```python
from build123d import *

# Parameters (mm, degrees)
SKETCH_1_R               = 150.987526818
SKETCH_1_R_2             = 138.21111966
EXTRUDE_1_DEPTH          = 15
FILLET_1_R               = 2
SKETCH_2_R               = 10
CUT_EXTRUDE_1_DEPTH      = 15
PATTERN_CIRCULAR_1_COUNT = 6


with BuildPart() as part:
    # Эскиз1 → Бобышка-Вытянуть1 (new body)
    with BuildSketch(Plane(origin=(0, 0, 0), x_dir=(1, 0, 0), z_dir=(0, 1, 0))):
        with Locations(Location((0, 0, 0), (0, 0, 270))):
            Circle(SKETCH_1_R)
        with Locations(Location((0, 0, 0), (0, 0, 270))):
            Circle(SKETCH_1_R_2, mode=Mode.SUBTRACT)
    extrude(amount=EXTRUDE_1_DEPTH)

    # Скругление1
    fillet_1_edges = [part.edges().sort_by_distance(p)[0] for p in [
        (0, 0, -150.987526818),
        (0, 0, -138.21111966),
    ]]
    fillet(fillet_1_edges, radius=FILLET_1_R)

    # Эскиз2 → Вырез-Вытянуть1 (cut)
    with BuildSketch(Plane(origin=(0, 0, 0), x_dir=(1, 0, 0), z_dir=(0, 1, 0))):
        with Locations((0, 150.987526818)):
            Circle(SKETCH_2_R)
    cut_extrude_1 = extrude(amount=CUT_EXTRUDE_1_DEPTH, mode=Mode.SUBTRACT)

    # Круговой массив1: Вырез-Вытянуть1 ×6 about axis
    pattern_circular_1_axis = Axis((0, 0, 0), (0, 1, 0))
    for i in range(1, PATTERN_CIRCULAR_1_COUNT):
        add(cut_extrude_1.rotate(pattern_circular_1_axis, i * 360 / PATTERN_CIRCULAR_1_COUNT), mode=Mode.SUBTRACT)


solid = part.part
```
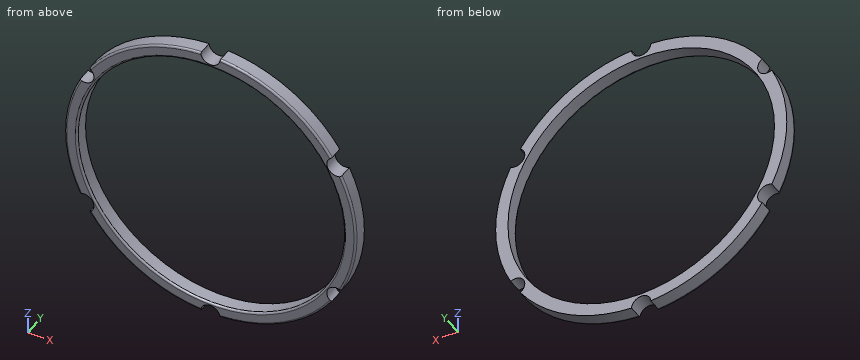
Read the model definition and answer for the solid it produces. Units are mm, in the model's axes. Give positions to 0.01 mm unless a question says otherwise; leave off trailing zeros. Write each loop counter-clockwise with the first axis right and the second up, starting at its lowest first coordinate (ties: lowest second). Pieces come first, ordered by that corner, then holes. Notation, with made-up numbers: (50, 46) - (66, 46) arc R29 ccw to (66, 83) - close; hole circle Ø6 at (19, -16.75). An arc over 180 degrees is marked (long way). Write item = value, one per line. Start each with the question number.
Item 1: Find section C-C (y = 11.5). Give the vertices of the cut face in (x, z), then the cut area to 3 significant figures.
Item 2: Find section B-B (x = 0). Give the vertices of the cut face in (y, z), then the cut area to 3 significant figures.
Item 3: Find section A-A (z = 0). Give the vertices of the cut face in (x, y), then the cut area to 3 significant figures.
Item 4: Each of these flat-tipped pins is pushed along its axis until it touches: P1, Ø2, axis at x = 42, y = 8.5, coming from the +Z side; P2, Ø1.5, axis at x = -59.5, y = 2.5, coming from the +Z side; P3, Ø5, axis at y = 2, z = -45.5, coming from the -X side. Where does it stop, or does it pass through?
Item 5: Find the intervals of material crossed by probe 1 along X at (y, z) = (5, -4); probe 2 along X at (y, z) = (6.25, 0); probe 3 along Z at (x, y) = (-63, 3.5), in increasing order. Write a range as [from, to].
Response:
q1.outline = (-135.47, -66.67) arc R10 cw to (-125.47, -83.98) arc R150.99 ccw to (-9.99, -150.66) arc R10 cw to (9.99, -150.66) arc R150.99 ccw to (125.47, -83.98) arc R10 cw to (135.47, -66.67) arc R150.99 ccw to (135.47, 66.67) arc R10 cw to (125.47, 83.98) arc R150.99 ccw to (9.99, 150.66) arc R10 cw to (-9.99, 150.66) arc R150.99 ccw to (-125.47, 83.98) arc R10 cw to (-135.47, 66.67) arc R150.99 ccw to start; hole circle Ø276.42 at (0, 0)
q1.area = 10,700 mm²
q2.outline = (0, -140.99) - (15, -140.99) - (15, -138.21) - (2, -138.21) arc R2 ccw to (0, -140.21) - close; (0, 140.21) arc R2 ccw to (2, 138.21) - (15, 138.21) - (15, 140.99) - (0, 140.99) - close
q2.area = 81.6 mm²
q3.outline = (-150.99, 2) arc R2 ccw to (-148.99, 0) - (-140.21, 0) arc R2 ccw to (-138.21, 2) - (-138.21, 15) - (-150.99, 15) - close; (138.21, 2) arc R2 ccw to (140.21, 0) - (148.99, 0) arc R2 ccw to (150.99, 2) - (150.99, 15) - (138.21, 15) - close
q3.area = 380 mm²
q4.P1 = 145.31
q4.P2 = 139.09
q4.P3 = -144.74
q5.probe_1 = [-150.93, -138.15], [138.15, 150.93]
q5.probe_2 = [-150.99, -138.21], [138.21, 150.99]
q5.probe_3 = [-137.22, -123.02], [123.02, 137.22]
